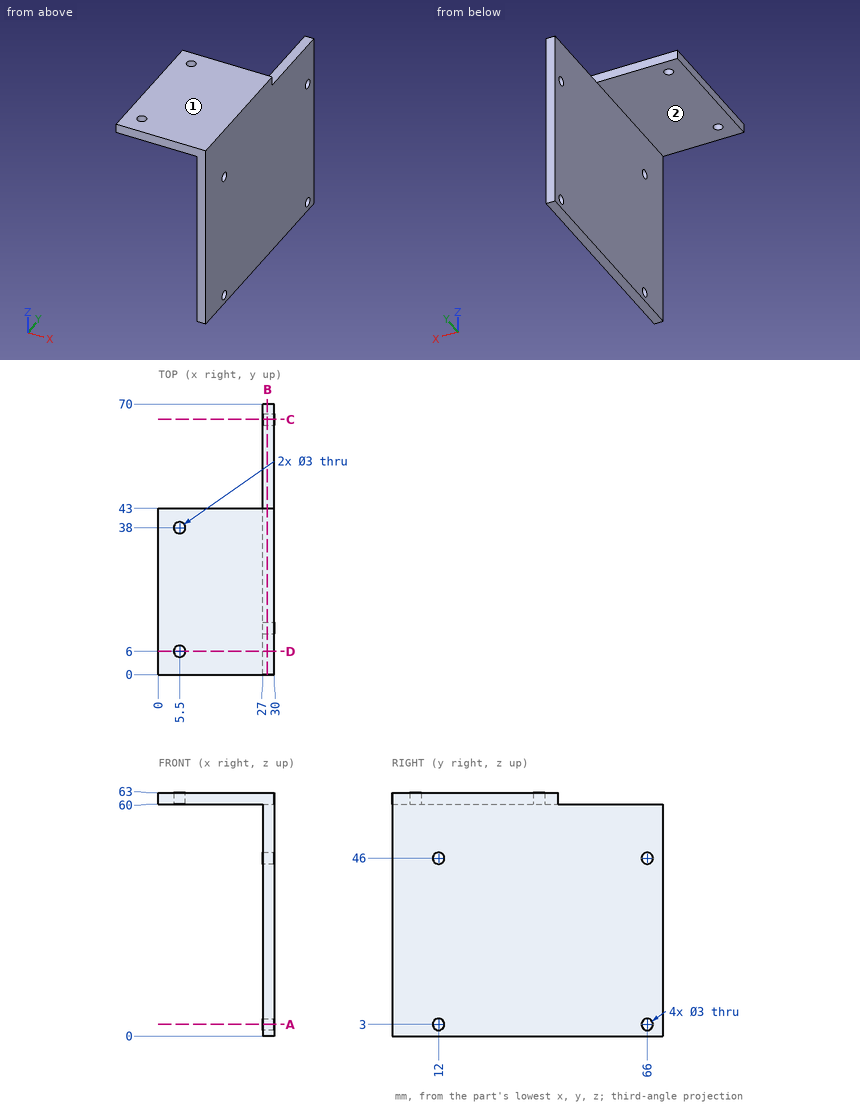
Part print with two shaded views. Sizes in mm from the minimum x, y, z corner. A direction names the side the tool comes from. Round coordinates to 2 decimals unless told otherwise and drop trailing zeros. Loops run counter-clockwise (first coordinate to the right, second up) from the corner with the lowest first, then second, coordinate; pieces in that order, holes last.
Item 1: Drill centre lines: line 1 along Y through (x, z) = (5.5, 61.55); line 2 along Y through (x, z) = (28.9, 46); line 3 along X through (y, z) = (32, 5). Where is each one in solid material? Low to high.
Item 2: Saw through at B-B (x = 28.25). List the corners of the cut face in (y, z), then the cut area to 3 significant figures.
Item 3: Which spindle directions (+Z, -Z, +X, -X, +Y, -Y) get a long thin tool onto all of the face, cutting with end or side? Do the marked faces 1 and 2. Say none if no direction does.
Item 4: Saw through at D-D (y = 6). List the corners of the cut face in (x, z), then the cut area to 3 significant figures.
Item 5: Saw through at C-C (y = 66). List the corners of the cut face in (x, z).
Item 6: Pin check, flat tips, straight feed: P1, Ø2.5, axis at x = 16.5, z = 61, coming from the +Y side; P2, Ø5, axis at y = 66, z = 46, coming from the -X side; P3, Ø13.5, axis at x = 13, y = 14.5, coming from the -Z side; P4, Ø12, axis at x = 17.5, y = 50.5, coming from the -Z side. Stop position of each tip, or through.
Item 7: Saw through at A-A (z = 3). List the corners of the cut face in (x, y).
Worked answers:
1. line 1: y = 0 to 4.5, 7.5 to 36.5, 39.5 to 43
1. line 2: y = 0 to 10.5, 13.5 to 64.5, 67.5 to 70
1. line 3: x = 27 to 30
2. outline: (0, 0) - (70, 0) - (70, 60) - (43, 60) - (43, 63) - (0, 63) - close; hole circle Ø3 at (12, 3); hole circle Ø3 at (12, 46); hole circle Ø3 at (66, 3); hole circle Ø3 at (66, 46)
2. area: 4,300 mm2
3. face 1: +Z, +X, -X, +Y, -Y
3. face 2: -Z, -X, +Y, -Y
4. outline: (0, 60) - (4, 60) - (4, 63) - (0, 63) - close; (7, 60) - (27, 60) - (27, 0) - (30, 0) - (30, 63) - (7, 63) - close
4. area: 261 mm2
5. outline: (27, 0) - (30, 0) - (30, 1.5) - (27, 1.5) - close; (27, 4.5) - (30, 4.5) - (30, 44.5) - (27, 44.5) - close; (27, 47.5) - (30, 47.5) - (30, 60) - (27, 60) - close
6. P1: stops at y = 43
6. P2: stops at x = 27
6. P3: stops at z = 60
6. P4: passes through
7. outline: (27, 0) - (30, 0) - (30, 10.5) - (27, 10.5) - close; (27, 13.5) - (30, 13.5) - (30, 64.5) - (27, 64.5) - close; (27, 67.5) - (30, 67.5) - (30, 70) - (27, 70) - close
